Check sheet for the drawn part. Datum: minimum x, y, z corner. Units: mm. Give positions to 0.01 mm unless a question says otherwise; leave off trailing zeros. Write each loop counter-clockwise with the first axis right and the second up, starting at its lowest first coordinate (ties: lowest second). Pieces come first, ordered by that corner, then holes. Notation, with made-up numbers: (65.25, 69.5) - (116.25, 69.5) arc R21 ccw to (116.25, 96.5) - close; hole circle Ø3 at (88, 18). An arc over 180 degrees is marked (long way). Use a Markdown table: item, result.
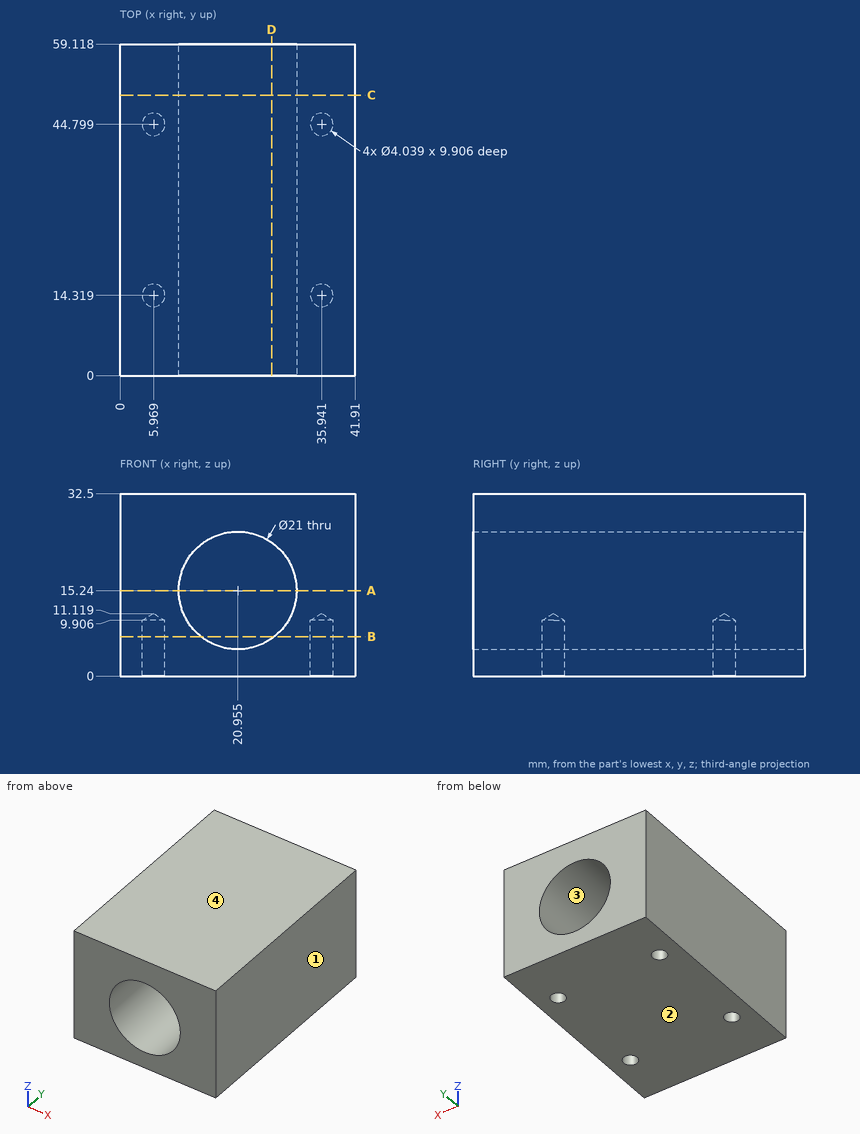
1) Section check A-A on z = 15.24. Record the boundary of the cut face in (x, y) (1 decimal), then the cut area to 3 significant figures.
Working result:
| item | result |
|---|---|
| outline | (0, 0) - (10.5, 0) - (10.5, 59.1) - (0, 59.1) - close; (31.5, 0) - (41.9, 0) - (41.9, 59.1) - (31.5, 59.1) - close |
| area | 1,240 mm² |
2) Depth check by flat-ended pin: P1, Ø3.5, axis at x = 35.94, y = 14.32, coming from the -Z side. Enter the tip coordinate at first touch or a pass-through.
Working result:
| item | result |
|---|---|
| P1 | stops at z = 10.07 |
3) Section check C-C on y = 50. Record the boundary of the cut face in (x, z) (1 decimal), then the cut area to 3 significant figures.
Working result:
| item | result |
|---|---|
| outline | (0, 0) - (41.9, 0) - (41.9, 32.5) - (0, 32.5) - close; hole circle Ø21 at (21, 15.2) |
| area | 1,020 mm² |
4) Section check D-D on x = 27. Record the boundary of the cut face in (y, z) (1 decimal).
Working result:
| item | result |
|---|---|
| outline | (0, 0) - (59.1, 0) - (59.1, 6.7) - (0, 6.7) - close; (0, 23.8) - (59.1, 23.8) - (59.1, 32.5) - (0, 32.5) - close |
5) Material ranges on L1, parallel to X at y = 23, z = 15; L2, parallel to Z at x = 21.5, y = 17.5 (1 decimal); L3, parallel to X at y = 43.5, z = 2 (1 decimal), recorded low to high. Write a range as from..to.
Working result:
| item | result |
|---|---|
| L1 | x = 0..10.46, 31.45..41.91 |
| L2 | z = 0..4.8, 25.7..32.5 |
| L3 | x = 0..4.4, 7.5..34.4, 37.5..41.9 |
6) Section check B-B on z = 7. Record the boundary of the cut face in (x, y), then the cut area to 3 significant figures.
Working result:
| item | result |
|---|---|
| outline | (0, 0) - (14.45, 0) - (14.45, 59.12) - (0, 59.12) - close; (27.46, 0) - (41.91, 0) - (41.91, 59.12) - (27.46, 59.12) - close; hole circle Ø4.04 at (5.97, 14.32); hole circle Ø4.04 at (5.97, 44.8); hole circle Ø4.04 at (35.94, 14.32); hole circle Ø4.04 at (35.94, 44.8) |
| area | 1,660 mm² |
7) Mould release check, pull along Z, two halves, no side actions. Record for the marked faces 1, 2, 3 and 4: pulls with the +Z half, pulls with the -Z half, needs draft (parallel to the pull), parting line crosses it, or undercut.
Working result:
| item | result |
|---|---|
| face 1 | needs draft |
| face 2 | pulls with the -Z half |
| face 3 | undercut |
| face 4 | pulls with the +Z half |
